Input: part model. Units: mm. Frame: model coordinates. Face numbers are marked on the shaded views. A direction names the side the tool comes from. Give positions to 0.01 mm unless a question says otherwise; leave off trailing zeros. Write each loop counter-clockwise with the first axis right and the second up, starting at its lowest first coordinate (ties: lowest second). Pieces come first, ordered by that corner, then holes.
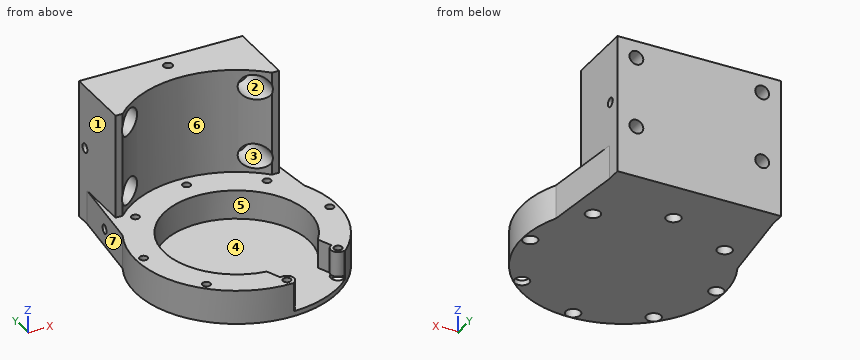
```python
from build123d import *

# Parameters (mm, degrees)
EXTRUDE_1_DEPTH          = 13.5
SKETCH_2_R               = 28.8
CUT_EXTRUDE_1_DEPTH      = 11.5
SKETCH_3_R               = 1.6
CUT_EXTRUDE_2_DEPTH      = 14.5
SKETCH_6_R               = 2.9
CUT_EXTRUDE_6_DEPTH      = 3.5
PATTERN_CIRCULAR_3_COUNT = 8
EXTRUDE_2_DEPTH          = 10
EXTRUDE_2_DEPTH_BACK     = 11
CUT_EXTRUDE_7_DEPTH      = 42.5
SKETCH_25_W              = 65
SKETCH_25_H              = 55
EXTRUDE_4_DEPTH          = 6
SKETCH_33_R              = 2.75
CUT_EXTRUDE_14_DEPTH     = 97
SKETCH_34_R              = 5
CUT_EXTRUDE_15_DEPTH     = 87
CUT_EXTRUDE_16_DEPTH     = 54.0000001
SKETCH_40_R              = 1.8
CUT_EXTRUDE_18_DEPTH     = 12
SKETCH_41_R              = 1.8
CUT_EXTRUDE_19_DEPTH     = 12
SKETCH_42_R              = 1.8
CUT_EXTRUDE_20_DEPTH     = 12
SKETCH_43_R              = 1.8
CUT_EXTRUDE_21_DEPTH     = 12


with BuildPart() as part:
    # Sketch 1 → Extrude 1 (new body)
    with BuildSketch(Plane.XY.offset(-14)):
        with BuildLine():
            Line((36.070726916, 17.288801572), (32.5, 50))
            Line((32.5, 50), (-32.5, 50))
            Line((-32.5, 50), (-36.070726916, 17.288801572))
            ThreePointArc((-36.070726916, 17.288801572), (0, -40), (36.070726916, 17.288801572))
        make_face()
    extrude(amount=-EXTRUDE_1_DEPTH)

    # Sketch 2 → Cut-Extrude 1 (cut)
    with BuildSketch(Plane.XY.offset(-14)):
        Circle(SKETCH_2_R)
    extrude(amount=-CUT_EXTRUDE_1_DEPTH, mode=Mode.SUBTRACT)

    # Sketch 3 → Cut-Extrude 2 (cut, through all)
    with BuildSketch(Plane(origin=(0, 0, -27.5), x_dir=(-1, 0, 0), z_dir=(0, 0, -1))):
        with Locations((0, 37)):
            Circle(SKETCH_3_R)
    cut_extrude_2 = extrude(amount=-CUT_EXTRUDE_2_DEPTH, mode=Mode.SUBTRACT)

    # Sketch 6 → Cut-Extrude 6 (cut)
    with BuildSketch(Plane(origin=(0, 0, -27.5), x_dir=(-1, 0, 0), z_dir=(0, 0, -1))):
        with Locations((0, 37)):
            Circle(SKETCH_6_R)
        with Locations((26.162950904, 26.162950904)):
            Circle(SKETCH_6_R)
        with Locations((37, 0)):
            Circle(SKETCH_6_R)
        with Locations((26.162950904, -26.162950904)):
            Circle(SKETCH_6_R)
        with Locations((-37, 0)):
            Circle(SKETCH_6_R)
        with Locations((-26.162950904, 26.162950904)):
            Circle(SKETCH_6_R)
        with Locations((0, -37)):
            Circle(SKETCH_6_R)
        with Locations((-26.162950904, -26.162950904)):
            Circle(SKETCH_6_R)
    extrude(amount=-CUT_EXTRUDE_6_DEPTH, mode=Mode.SUBTRACT)

    # Pattern Circular 3: Cut-Extrude 2 ×8 about axis
    pattern_circular_3_axis = Axis((0, 0, 0), (0, 0, 1))
    for i in range(1, PATTERN_CIRCULAR_3_COUNT):
        add(cut_extrude_2.rotate(pattern_circular_3_axis, i * 360 / PATTERN_CIRCULAR_3_COUNT), mode=Mode.SUBTRACT)



with BuildPart() as body_2:
    # Sketch 7 → Extrude 2 (new body, two sides)
    with BuildSketch(Plane(origin=(0, 40, 0), x_dir=(1, 0, 0), z_dir=(0, 1, 0))) as extrude_2_sk:
        Polygon((-32.5, 0), (-32.5, 16.283385264), (-32.5, 27.5), (-5.850968587, 27.5), (-5.850968587, 14), (5.653955786, 14), (5.653955786, 27.5), (32.5, 27.5), (32.5, 16.283385264), (32.5, 0), (32.5, -27.5), (0, -27.5), (-32.5, -27.5), align=None)
    extrude(amount=EXTRUDE_2_DEPTH)
    extrude(extrude_2_sk.sketch, amount=-EXTRUDE_2_DEPTH_BACK)

    # Sketch 9 → Cut-Extrude 7 (cut, through all)
    with BuildSketch(Plane.XY.offset(-14)):
        with BuildLine():
            Line((-31.306275756, 27.242743956), (31.306275756, 27.242743956))
            ThreePointArc((31.306275756, 27.242743956), (0, 41.5), (-31.306275756, 27.242743956))
        make_face()
    extrude(amount=CUT_EXTRUDE_7_DEPTH, mode=Mode.SUBTRACT)


with BuildPart() as part_1:
    add(part.part)

    add(body_2.part)  # Extrude 4 merges body 2
    # Sketch 25 → Extrude 4 (add)
    with BuildSketch(Plane(origin=(0, 50, 0), x_dir=(1, 0, 0), z_dir=(0, 1, 0))):
        Rectangle(SKETCH_25_W, SKETCH_25_H)
    extrude(amount=EXTRUDE_4_DEPTH)

    # Sketch 33 → Cut-Extrude 14 (cut, through all)
    with BuildSketch(Plane(origin=(0, 56, 0), x_dir=(1, 0, 0), z_dir=(0, 1, 0))):
        with Locations((-25, 7.25)):
            Circle(SKETCH_33_R)
        with Locations((25, 7.25)):
            Circle(SKETCH_33_R)
        with Locations((-25, -20.75)):
            Circle(SKETCH_33_R)
        with Locations((25, -20.75)):
            Circle(SKETCH_33_R)
    extrude(amount=-CUT_EXTRUDE_14_DEPTH, mode=Mode.SUBTRACT)

    # Sketch 34 → Cut-Extrude 15 (cut, through all)
    with BuildSketch(Plane(origin=(0, 46, 0), x_dir=(1, 0, 0), z_dir=(0, 1, 0))):
        with Locations((-25, 7.25)):
            Circle(SKETCH_34_R)
        with Locations((25, 7.25)):
            Circle(SKETCH_34_R)
        with Locations((-25, -20.75)):
            Circle(SKETCH_34_R)
        with Locations((25, -20.75)):
            Circle(SKETCH_34_R)
    extrude(amount=-CUT_EXTRUDE_15_DEPTH, mode=Mode.SUBTRACT)

    # Sketch 35 → Cut-Extrude 16 (cut, through all)
    with BuildSketch(Plane.XY.offset(-25.5)):
        with BuildLine():
            Line((-5.482310635, -23.69583549), (20.700351605, -12.906620763))
            Line((20.700351605, -12.906620763), (25.058065646, -23.48167722))
            ThreePointArc((25.058065646, -23.48167722), (23.48167722, -27.267836162), (27.267836162, -28.844224588))
            Line((27.267836162, -28.844224588), (28.638176696, -32.169690276))
            Line((28.638176696, -32.169690276), (2.465370124, -42.982822188))
            Line((2.465370124, -42.982822188), (1.104885258, -39.681273684))
            ThreePointArc((1.104885258, -39.681273684), (2.681273684, -35.895114742), (-1.104885258, -34.318726316))
            Line((-1.104885258, -34.318726316), (-5.482310635, -23.69583549))
        make_face()
    extrude(amount=CUT_EXTRUDE_16_DEPTH, mode=Mode.SUBTRACT)

    # Sketch 40 → Cut-Extrude 18 (cut)
    with BuildSketch(Plane.XY.offset(27.5)):
        with Locations((0, 50.608642373)):
            Circle(SKETCH_40_R)
    extrude(amount=-CUT_EXTRUDE_18_DEPTH, mode=Mode.SUBTRACT)

    # Sketch 41 → Cut-Extrude 19 (cut)
    with BuildSketch(Plane(origin=(-37.510987458, 4.09466785, 0), x_dir=(0, 0, 1), z_dir=(-0.99409486, 0.108514559, 0))):
        with Locations((-20.75, 29.979930787)):
            Circle(SKETCH_41_R)
    extrude(amount=-CUT_EXTRUDE_19_DEPTH, mode=Mode.SUBTRACT)

    # Sketch 42 → Cut-Extrude 20 (cut)
    with BuildSketch(Plane(origin=(32.5, 0, 0), x_dir=(0, 0, -1), z_dir=(1, 0, 0))):
        with Locations((-3.254490718, 50.718137082)):
            Circle(SKETCH_42_R)
    extrude(amount=-CUT_EXTRUDE_20_DEPTH, mode=Mode.SUBTRACT)

    # Sketch 43 → Cut-Extrude 21 (cut)
    with BuildSketch(Plane.ZY.offset(32.5)):
        with Locations((2.489697323, 51.600552718)):
            Circle(SKETCH_43_R)
    extrude(amount=-CUT_EXTRUDE_21_DEPTH, mode=Mode.SUBTRACT)


solid = part_1.part
```
Q1. Section B-B, the plane z = -7.25. Return the cut outline in (x, y), then the cut area to 3 significant figures.
Q2. Access query for the marked faces 5, 6 and 7. Directions: +Z, -Z, +X, -X, +Y, -Y. A direction counts if a zero-diameter tool reaches every point of the face in a straight line with its end or side. Return the directions, or none.
Q3. Material intervals for line 1 along Z through (x, y) = (25, 38); line 2 along Z through (x, y) = (-25, 51.5); line 3 along X through (y, z) = (53.5, -7.25), sorted ascending.
Q4. Mould query, pull axis Z, two halves, no side actions, for the marked faces 1, 2, 3 and 4. Classes: +Z half, -Z half, draft (parallel to the pull), parting line (faces both ways), or undercut.
Q5. Section D-D, the plane z = 13.5. Return the cut outline in (x, y), then the cut area to 3 significant figures.
Q6. Section A-A, the plane x = 0. Give the number of separate pieces and of enclosed holes in the cut face, then the cut area to 3 significant figures.
Q7. Pin query (flat end, axial travel): pin 1 (12 mm diameter, centred on x = 16.5, z = -9.5, fed in from -Y); pin 2 (8 mm diameter, centred on x = 0.5, z = 5, fed in from -Y); pin 3 (3 mm diameter, centred on x = 25, z = 18.5, fed in from -Y); pin 4 (3.5 mm diameter, centred on x = 25, z = 20.75, fed in from -Y). Return the tip coordinate at first contact, or that it passes through.
Q8. Section C-C, the plane y = -8.5. Return the cut outline in (x, z), then the cut area to 3 significant figures.
Solutions:
1. outline: (-32.5, 29) - (-30, 29) - (-30, 46) - (-27.75, 46) - (-27.75, 56) - (-32.5, 56) - close; (-22.25, 46) - (-20, 46) - (-20, 36.36) arc R41.5 cw to (20, 36.36) - (20, 46) - (22.25, 46) - (22.25, 56) - (-22.25, 56) - close; (27.75, 46) - (30, 46) - (30, 29) - (32.5, 29) - (32.5, 56) - (27.75, 56) - close
1. area: 872 mm2
2. face 5: +Z
2. face 6: +Z, -Y
2. face 7: +Z, -Z, -X, +Y
3. line 1: z = -27.5 to -12.25, -2.25 to 15.75, 25.75 to 27.5
3. line 2: z = -27.5 to -10, -4.5 to 0.69, 4.29 to 18, 23.5 to 27.5
3. line 3: x = -32.5 to -27.75, -22.25 to 22.25, 27.75 to 32.5
4. face 1: draft
4. face 2: undercut
4. face 3: undercut
4. face 4: +Z half
5. outline: (-32.5, 29) - (-29.69, 29) arc R41.5 cw to (29.69, 29) - (32.5, 29) - (32.5, 56) - (-32.5, 56) - close
5. area: 1,240 mm2
6. separate pieces: 4
6. enclosed holes: 0
6. area: 1,030 mm2
7. pin 1: stops at y = 20.26
7. pin 2: stops at y = 41.26
7. pin 3: stops at y = 46
7. pin 4: passes through
8. outline: (-39.09, -27.5) - (39.09, -27.5) - (39.09, -14) - (27.52, -14) - (27.52, -25.5) - (-27.52, -25.5) - (-27.52, -14) - (-39.09, -14) - close
8. area: 422 mm2
